Part model, mm, in its own coordinate system. A direction names the side the tool comes from. Coordinates: 2 decimals unless noted, no trailing zeros. Write each loop counter-clockwise with the first axis right and the second up, starting at its lowest first coordinate (ties: lowest second). Pieces come first, ordered by that corner, then holes. Notation, with made-up numbers: M -22,10 L 1,10 A21 cw 1,40 Z; hole C -22.75,64.25 d6. An arc over 180 degrees is marked long. Use a Markdown table: item, result. Add a question column.
Q1. Slice it at C-C on z = -12.5. Write the cut outline in (x, y), then the cut area to 3 significant figures.
Q2. Tool access for faces 4 (the flat face through (7, -1, -32.151)), 5 (the cylindrical face through (-7.485, -33.708, -8.198)), 6 (the flat face through (-55.761, -1, -25)): list every direction of +Z, -Z, +X, -X, +Y, -Y with a clear straight run to the whole face (end or side of a thin tool).
Q3. Slice it at A-A on y = 0. Write the cut outline in (x, z), then the cut area to 3 significant figures.
Q4. Slice it at B-B on x = 0. Write the cut outline in (y, z), then the cut area to 3 significant figures.
Q5. Slice it at D-D on x = -31.5. Write the cut outline in (y, z), then the cut area to 3 significant figures.
Q6. Wall check: L1, parallel to Z at x = 43, y = 22; L2, parallel to Y at x = 0, z = -8.25; L3, parallel to Z at x = 5, y = 24.5. Give the ranges that are in metal, low to high. Write a range as from..to.
Q7. Mould opens along Z. For faces 1 (the flat face through (-38, 1, 0)), 2 (the flat face through (39, -1, -16.63)), 3 (the flat face through (55.761, -1, -41)) say: released by +Z, released by -Z, zero draft, split by the parting line, or undercut.
from build123d import *

# Parameters (mm, degrees)
F0_W     = 111.522756
F0_H     = 86.371966
F1_DEPTH = 50.8
F2_W     = 80.143302
F2_H     = 39.228082
F3_DEPTH = 36.405057
F4_W     = 96.042376
F4_H     = 15.521109
F5_DEPTH = 86.372966
F6_R     = 34.528896
F7_DEPTH = 25.4


with BuildPart() as f1:
    # F0 (on Top) → F1 (new body)
    with BuildSketch(Plane.XY):
        Rectangle(F0_W, F0_H)
    extrude(amount=-F1_DEPTH)

    # F2 (on face) → F3 (join)
    with BuildSketch(Plane.XZ.offset(43.185983)):
        with Locations((0, -31.185959)):
            Rectangle(F2_W, F2_H)
    extrude(amount=-F3_DEPTH)

    # F4 (on face) → F5 (cut, through all)
    with BuildSketch(Plane.XZ.offset(43.185983)):
        with Locations((7.74019, -24.390307)):
            Rectangle(F4_W, F4_H)
    extrude(amount=-F5_DEPTH, mode=Mode.SUBTRACT)

    # F6 (on face) → F7 (cut)
    with BuildSketch(Plane.XY):
        Circle(F6_R)
    extrude(amount=-F7_DEPTH, mode=Mode.SUBTRACT)


solid = f1.part
Recorded:
| question | item | result |
|---|---|---|
| 1 | outline | M -55.76,-43.19 L 55.76,-43.19 L 55.76,43.19 L -55.76,43.19 Z; hole C 0,0 d69.06 |
| 1 | area | 5,890 mm² |
| 2 | face 4 | +X, +Y, -Y |
| 2 | face 5 | +Z |
| 2 | face 6 | +Z, -Z, -X, +Y, -Y |
| 3 | outline | M -55.76,-50.8 L 55.76,-50.8 L 55.76,-32.15 L -40.28,-32.15 L -40.28,-16.63 L -34.53,-16.63 L -34.53,0 L -55.76,0 Z; M 34.53,-16.63 L 55.76,-16.63 L 55.76,0 L 34.53,0 Z |
| 3 | area | 3,030 mm² |
| 4 | outline | M -43.19,-50.8 L 43.19,-50.8 L 43.19,-32.15 L -43.19,-32.15 Z; M -43.19,-16.63 L -34.53,-16.63 L -34.53,0 L -43.19,0 Z; M 34.53,-16.63 L 43.19,-16.63 L 43.19,0 L 34.53,0 Z |
| 4 | area | 1,900 mm² |
| 5 | outline | M -43.19,-50.8 L 43.19,-50.8 L 43.19,-32.15 L -43.19,-32.15 Z; M -43.19,-16.63 L -14.14,-16.63 L -14.14,0 L -43.19,0 Z; M 14.14,-16.63 L 43.19,-16.63 L 43.19,0 L 14.14,0 Z |
| 5 | area | 2,580 mm² |
| 6 | L1 | -50.8..-32.15, -16.63..0 |
| 6 | L2 | -43.19..-34.53, 34.53..43.19 |
| 6 | L3 | -50.8..-32.15 |
| 7 | face 1 | released by +Z |
| 7 | face 2 | undercut |
| 7 | face 3 | zero draft |
